```python
from build123d import *

# Parameters (mm, degrees)
F0_R     = 13.5
F0_R_2   = 12
F1_DEPTH = 12.75
F2_SIZE2 = 0.5773502692
F2_SIZE  = 1
F3_R     = 2.5
F4_DEPTH = 13.501


with BuildPart() as f1:
    # F0 (on Front) → F1 (new body, symmetric)
    with BuildSketch(Plane.XZ):
        Circle(F0_R)
        Circle(F0_R_2, mode=Mode.SUBTRACT)
    extrude(amount=F1_DEPTH, both=True)

    # F2
    f2_edges = [f1.edges().sort_by_distance(p)[0] for p in [
        (-12, -12.75, 0),
        (-12, 12.75, 0),
    ]]
    f2_side = f1.faces().sort_by_distance((-12, 0, 0))[0]
    chamfer(f2_edges, length=F2_SIZE, length2=F2_SIZE2, reference=f2_side)

    # F3 (on Top) → F4 (cut, through all)
    with BuildSketch(Plane.XY):
        Circle(F3_R)
    extrude(amount=F4_DEPTH, mode=Mode.SUBTRACT)


solid = f1.part
```
The model under review builds one solid part; all positions refer to its coordinate system, in mm. A direction names the side the tool comes from. Give positions to 0.01 mm unless a question says otherwise; leave off trailing zeros. Write each loop counter-clockwise with the first axis right and the second up, starting at its lowest first coordinate (ties: lowest second). Pieces come first, ordered by that corner, then holes. Notation, with made-up numbers: (51, 28.5) - (75, 28.5) arc R17 ccw to (75, 59.5) - close; hole circle Ø6 at (-25.75, 16.5). An arc over 180 degrees is marked (long way). Answer in a Markdown table with one row per item. Add a question column.
1. Draft analysis for pull direction Z (two halves, no side actions). For faces 3 (the flat face through (9, 12.75, -9)), 4 (the cylindrical face through (-2.601, 0.165, -11.715)), 5 (the cylindrical face through (-2.93, -0.18, -13.18)), state which applies: +Z half, -Z half, draft (parallel to the pull), parting line (faces both ways), or undercut.
2. Tool access review of faces 1 (the cylindrical face through (2.385, 0.751, 12.606)), 2 (the flat face through (9, -12.75, -9)): name each direction out of +Z, -Z, +X, -X, +Y, -Y from which nothing blocks a thin tool from reaching the whole face with its end or side.
3. We need section C-C on y = -5. Write out the cut boundary in (x, z).
4. Insertion check: P1, Ø4, axis at x = -5.5, y = 5.5, coming from the +Z side; P2, Ø12, axis at x = -4, z = -0.5, coming from the -Y side; P3, Ø1, axis at y = 5, z = 6.5, coming from the +X side; P4, Ø2, axis at x = -6.5, y = 6, coming from the -Z side. Each pin has a flat end and moves straight along its axis. Give the tip position at first contact, or say it passes through.
5. We need section D-D on y = 0. Write out the cut boundary in (x, z), then the cut area to 3 significant figures.
6. We need section A-A on x = 0. Write out the cut boundary in (y, z), then the cut area to 3 significant figures.
7. We need section B-B on z = 0. Write out the cut boundary in (x, y).
8. Wall thickness on line 1 along Z through (x, y) = (0, 3.75); line 2 along Y through (x, z) = (0, 12.6); line 3 along Z through (x, y) = (3.75, 3.5): over which ranges is each line inside the solid? List them lowest first. Write a range as [from, to].
Ans:
| question | item | result |
|---|---|---|
| 1 | face 3 | draft |
| 1 | face 4 | undercut |
| 1 | face 5 | parting line |
| 2 | face 1 | +Z |
| 2 | face 2 | +Z, -Z, +X, -X, -Y |
| 3 | outline | circle Ø27 at (0, 0); hole circle Ø24 at (0, 0) |
| 4 | P1 | stops at z = 13.04 |
| 4 | P2 | passes through |
| 4 | P3 | stops at x = 12.09 |
| 4 | P4 | stops at z = -12.33 |
| 5 | outline | (-2.5, 11.74) - (-2.5, 13.27) arc R13.5 ccw (long way) to (2.5, 13.27) - (2.5, 11.74) arc R12 cw (long way) to start |
| 5 | area | 113 mm^2 |
| 6 | outline | (-12.75, -13.5) - (12.75, -13.5) - (12.75, -12.58) - (11.75, -12) - (-11.75, -12) - (-12.75, -12.58) - close; (-12.75, 12.58) - (-11.75, 12) - (-2.5, 12) - (-2.5, 13.5) - (-12.75, 13.5) - close; (2.5, 12) - (11.75, 12) - (12.75, 12.58) - (12.75, 13.5) - (2.5, 13.5) - close |
| 6 | area | 67.8 mm^2 |
| 7 | outline | (-13.5, -12.75) - (-12.58, -12.75) - (-12, -11.75) - (-12, 11.75) - (-12.58, 12.75) - (-13.5, 12.75) - close; (12, -11.75) - (12.58, -12.75) - (13.5, -12.75) - (13.5, 12.75) - (12.58, 12.75) - (12, 11.75) - close |
| 8 | line 1 | z = [-13.5, -12], [12, 13.5] |
| 8 | line 2 | y = [-12.75, -2.5], [2.5, 12.75] |
| 8 | line 3 | z = [-12.97, -11.4], [11.4, 12.97] |
